```python
from build123d import *

# Parameters (mm, degrees)
F1_DEPTH = 60
F0_W     = 10
F0_H     = 20
F2_DEPTH = 2
F3_SIZE  = 10


with BuildPart() as f1:
    # F0 (on Top) → F1 (new body)
    with BuildSketch(Plane.XY):
        Polygon((-19.530129, -10.959504), (-19.530129, 9.040496), (-9.530129, 9.040496), (13.469871, 9.040496), (23.469871, 9.040496), (23.469871, -10.959504), (13.469871, -10.959504), (13.469871, -12.959504), (25.469871, -12.959504), (25.469871, 11.040496), (-21.530129, 11.040496), (-21.530129, -12.959504), (-9.530129, -12.959504), (-9.530129, -10.959504), align=None)
    extrude(amount=F1_DEPTH)

    # F0 (on Top) → F2 (join)
    with BuildSketch(Plane.XY):
        with Locations((-14.530129, -0.959504)):
            Rectangle(F0_W, F0_H)
        with Locations((18.469871, -0.959504)):
            Rectangle(F0_W, F0_H)
    extrude(amount=F2_DEPTH)

    # F3
    f3_edges = [f1.edges().sort_by_distance(p)[0] for p in [
        (-9.530129, -11.959504, 60),
        (13.469871, -11.959504, 60),
    ]]
    chamfer(f3_edges, length=F3_SIZE)


solid = f1.part
```
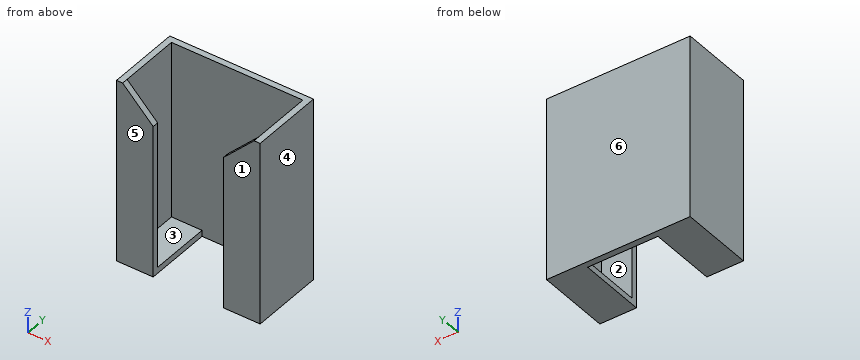
For this review, take the finished solid that the model builds, in its own axes (mm). Face numbers are marked on the shaded views. A direction names the side the tool comes from. Round coordinates to 2 decimals unless told otherwise and drop trailing zeros. Write each loop counter-clockwise with the first axis right and the second up, starting at its lowest first coordinate (ties: lowest second). Pieces come first, ordered by that corner, then holes. Notation, with made-up numbers: (69, 9.5) -> (127, 9.5) arc R13 cw to (127, 23.5) -> close; hole circle Ø10 at (60, 81.25). An arc over 180 degrees is marked (long way). One line per question, with ' | ' between items. Start each with the question number.
(1) For line 1 along X through (y, z) = (-1.5, 48.5); line 2 along Y through (x, z) = (-17, 35); line 3 along X through (y, z) = (-11.5, 40), list the stretches that pass through material, from the lowest coordinate up. Write a range as from..to.
(2) Tool access review of the marked faces 1 and 2: name each direction out of +Z, -Z, +X, -X, +Y, -Y from which nothing blocks a thin tool from reaching the whole face with its end or side.
(3) Mouldability with a two-part tool opening along Y and no side actions: class the marked faces 3, 4, 5 and 6 as released by +Y, released by -Y, zero draft, split by the parting line, or undercut.
(4) Add section B-B, the plane z = 30. Write out the cut boundary in (x, y), plus the area to 3 significant figures.
(5) Add section C-C, the plane x = -16. Write out the cut boundary in (y, z), plus the area to 3 significant figures.
(6) Insertion check: P1, Ø4, axis at x = -8.5, y = -6, coming from the +Z side; P2, Ø6, axis at x = 14.5, y = -8.5, coming from the +Z side; P3, Ø8, axis at x = 2.5, z = 33.5, coming from the -Y side; P4, Ø6, axis at x = 0.5, y = 6, coming from the +Z side. Each pin has a flat end and moves straight along its axis. Give the tip position at first contact, or say it passes through.
(7) Add section A-A, the plane y = -6.75. Write out the cut boundary in (x, z).
(8) Add section D-D, the plane x = 19.5. Write out the cut boundary in (y, z), plus the area to 3 significant figures.
Answer list:
1) line 1: -21.53..-19.53, 23.47..25.47 | line 2: -12.96..-10.96, 9.04..11.04 | line 3: -21.53..-9.53, 13.47..25.47
2) face 1: +Z, -Z, +X, -X, -Y | face 2: +Z
3) face 3: undercut | face 4: zero draft | face 5: released by -Y | face 6: released by +Y
4) outline: (-21.53, -12.96) -> (-9.53, -12.96) -> (-9.53, -10.96) -> (-19.53, -10.96) -> (-19.53, 9.04) -> (23.47, 9.04) -> (23.47, -10.96) -> (13.47, -10.96) -> (13.47, -12.96) -> (25.47, -12.96) -> (25.47, 11.04) -> (-21.53, 11.04) -> close | area: 222 mm²
5) outline: (-12.96, 0) -> (11.04, 0) -> (11.04, 60) -> (9.04, 60) -> (9.04, 2) -> (-10.96, 2) -> (-10.96, 56.47) -> (-12.96, 56.47) -> close | area: 273 mm²
6) P1: z = 2 | P2: z = 52.75 | P3: y = 9.04 | P4: through
7) outline: (-21.53, 0) -> (-9.53, 0) -> (-9.53, 2) -> (-19.53, 2) -> (-19.53, 60) -> (-21.53, 60) -> close; (13.47, 0) -> (25.47, 0) -> (25.47, 60) -> (23.47, 60) -> (23.47, 2) -> (13.47, 2) -> close
8) outline: (-12.96, 0) -> (11.04, 0) -> (11.04, 60) -> (9.04, 60) -> (9.04, 2) -> (-10.96, 2) -> (-10.96, 56.03) -> (-12.96, 56.03) -> close | area: 272 mm²
